Could you check a few things on this model? Use its own coordinates, in mm. Face numbers are marked on the shaded views. A direction names the side the tool comes from. Coordinates: 2 decimals unless noted, no trailing zeros. Write each loop counter-clockwise with the first axis right and the second up, starting at its lowest first coordinate (ties: lowest second). Pieces come first, ordered by that corner, then holes.
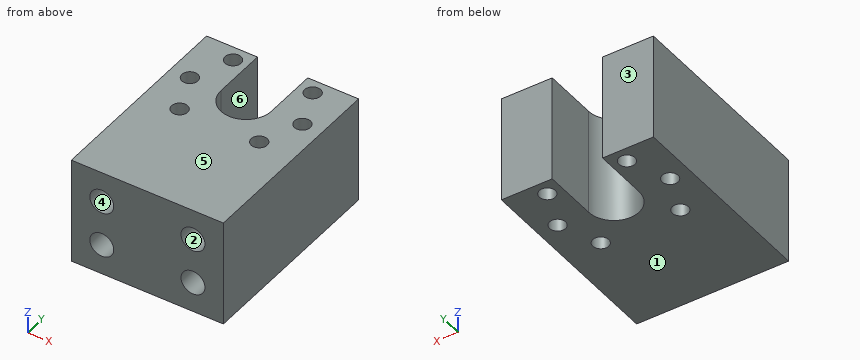
```python
from build123d import *

# Parameters (mm, degrees)
F0_W     = 63.5
F0_H     = 44.45
F1_DEPTH = 84.1375
F2_R     = 5
F3_DEPTH = 25.4
F4_R     = 3.35
F5_DEPTH = 44.451


with BuildPart() as f1:
    # F0 (on Front) → F1 (new body)
    with BuildSketch(Plane.XZ):
        with Locations((-33.239908, 2.843605)):
            Rectangle(F0_W, F0_H)
    extrude(amount=F1_DEPTH)

    # F2 (on face) → F3 (cut)
    with BuildSketch(Plane.XZ.offset(84.1375)):
        with Locations((-52.289908, 12.368605)):
            Circle(F2_R)
        with Locations((-52.289908, -6.681395)):
            Circle(F2_R)
        with Locations((-14.189908, 12.368605)):
            Circle(F2_R)
        with Locations((-14.189908, -6.681395)):
            Circle(F2_R)
    extrude(amount=-F3_DEPTH, mode=Mode.SUBTRACT)

    # F4 (on face) → F5 (cut, through all)
    with BuildSketch(Plane(origin=(0, 0, -19.381395), x_dir=(1, 0, 0), z_dir=(0, 0, -1))):
        with Locations((-56.739908, 22.688)):
            Circle(F4_R)
        with Locations((-49.856917, 6.070991)):
            Circle(F4_R)
        with Locations((-16.622898, 6.070991)):
            Circle(F4_R)
        with Locations((-9.739908, 22.688)):
            Circle(F4_R)
        with Locations((-16.622898, 39.305009)):
            Circle(F4_R)
        with Locations((-49.856917, 39.305009)):
            Circle(F4_R)
        with BuildLine():
            Line((-22.739908, 0), (-22.739908, 22.688))
            ThreePointArc((-22.739908, 22.688), (-33.239908, 33.188), (-43.739908, 22.688))
            Line((-43.739908, 22.688), (-43.739908, 0))
            Line((-43.739908, 0), (-22.739908, 0))
        make_face()
    extrude(amount=-F5_DEPTH, mode=Mode.SUBTRACT)


solid = f1.part
```
1. On a 3-axis mill with a long thin cutter (end or side, diameter ignored), from which of +Z, -Z, +X, -X, +Y, -Y can I reach the whole of each face in a straight line? I mean the marked faces 4, 5 and 6. Say none if no direction works.
Verdict:
face 4: -Y
face 5: +Z, +X, -X, +Y, -Y
face 6: +Z, -Z, +Y
2. I want a section at B-B on z = -8. Give the number of separate pieces and of enclosed holes in the cut face, plus the area to 3 significant figures.
Verdict:
separate pieces: 1
enclosed holes: 6
area: 3,990 mm2
3. For pin 1 (5 mm diameter, centred on x = -51, z = 10.5, fed in from -Y), with a flat end and sliding along its axis, tell me the tip position at first contact or that it passes through.
Verdict:
pin 1: stops at y = -58.74
4. Please list where these lines run through material, in increasing order: line 1 along X through (y, z) = (-38.5, -2); line 2 along X through (y, z) = (-24, 8); line 3 along Y through (x, z) = (-14, 12).
Verdict:
line 1: x = -64.99 to -53.11, -46.61 to -19.87, -13.37 to -1.49
line 2: x = -64.99 to -59.82, -53.66 to -43.66, -22.82 to -12.82, -6.66 to -1.49
line 3: y = -58.74 to -41.39, -37.22 to -8.15, -3.99 to 0
5. I want a section at A-A on y = -13. Please give me the cut outline in (x, z).
Verdict:
outline: (-64.99, -19.38) - (-43.74, -19.38) - (-43.74, 25.07) - (-64.99, 25.07) - close; (-22.74, -19.38) - (-1.49, -19.38) - (-1.49, 25.07) - (-22.74, 25.07) - close
6. I want a section at D-D on y = -38. Please give me the cut outline in (x, z).
Verdict:
outline: (-64.99, -19.38) - (-52.94, -19.38) - (-52.94, 25.07) - (-64.99, 25.07) - close; (-46.77, -19.38) - (-19.71, -19.38) - (-19.71, 25.07) - (-46.77, 25.07) - close; (-13.54, -19.38) - (-1.49, -19.38) - (-1.49, 25.07) - (-13.54, 25.07) - close
7. I want a section at C-C on x = -15. Please give me the cut outline in (y, z).
Verdict:
outline: (-84.14, -19.38) - (-42.24, -19.38) - (-42.24, 25.07) - (-84.14, 25.07) - (-84.14, 17.3) - (-58.74, 17.3) - (-58.74, 7.43) - (-84.14, 7.43) - (-84.14, -1.75) - (-58.74, -1.75) - (-58.74, -11.62) - (-84.14, -11.62) - close; (-36.37, -19.38) - (-9, -19.38) - (-9, 25.07) - (-36.37, 25.07) - close; (-3.14, -19.38) - (0, -19.38) - (0, 25.07) - (-3.14, 25.07) - close
8. If we mould it in two halves opening along Z, with no side actions, what happens to the marked faces 1, 2 and 3? For each: pulls with the +Z half, pulls with the -Z half, needs draft (parallel to the pull), parting line crosses it, or undercut.
Verdict:
face 1: pulls with the -Z half
face 2: undercut
face 3: needs draft
